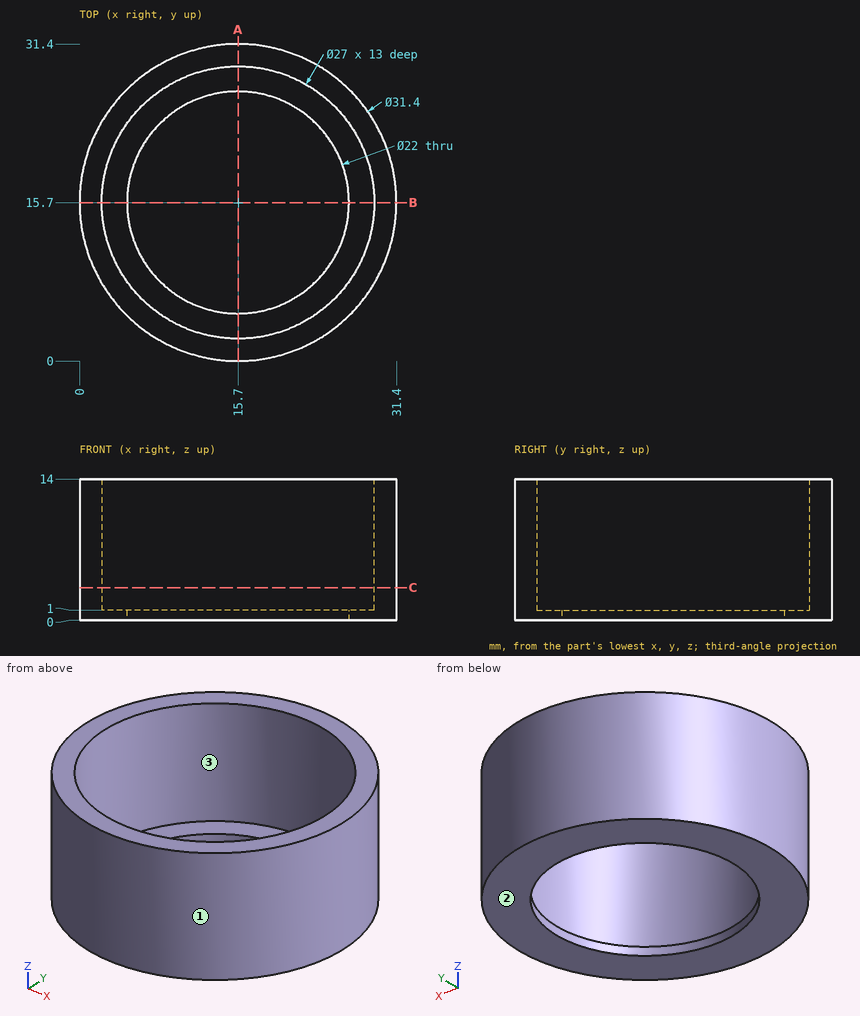
Job drawing, mm, ordinate dimensions from the low corner. One solid piece. Give positions to 0.01 mm unless a question says otherwise; leave off trailing zeros. Order: outer loops, then holes, each group sorted by start corner. A loop starts at its lowest first (then second) coordinate and runs counter-clockwise, first axis right, second up. Notation, with made-up numbers: (29, 10) - (62, 10) arc R15 ccw to (62, 17) - close; hole circle Ø4 at (68, -7). An arc over 180 degrees is marked (long way). Return JSON: item names as keys, results as strings.
1) Cut at C-C, the plane z = 3.25. Give the cut face in (x, y), plus the area to 3 significant figures.
Geometry says:
{"outline": "circle Ø31.4 at (15.7, 15.7); hole circle Ø27 at (15.7, 15.7)", "area": "202 mm²"}
2) Cut at A-A, the plane x = 15.7. Give the cut face in (y, z).
Geometry says:
{"outline": "(0, 0) - (4.7, 0) - (4.7, 1) - (2.2, 1) - (2.2, 14) - (0, 14) - close; (26.7, 0) - (31.4, 0) - (31.4, 14) - (29.2, 14) - (29.2, 1) - (26.7, 1) - close"}
3) Probe line 1 (Y direction, x = 15.7, z = 0.2); line 2 (X direction, y = 16, z = 1.25); line 3 (Y direction, x = 24, z = 13). List the from-to ranges inside material, lowest first. Write a range as from..to.
Geometry says:
{"line 1": "0..4.7, 26.7..31.4", "line 2": "0..2.2, 29.2..31.4", "line 3": "2.37..5.05, 26.35..29.03"}
4) Flat gauge pins, fed straight in: P1, Ø1, axis at x = 6, z = 2, coming from the +Y side; P2, Ø3, axis at x = 18, z = 7.5, coming from the +Y side; P3, Ø3, axis at x = 3.5, z = 2.5, coming from the +Y side. Where does each tip first touch, or does it go through?
Geometry says:
{"P1": "y = 28.42", "P2": "y = 31.38", "P3": "y = 27.19"}
5) Pull direction Y, two halves, no side cores. Call the marked faces 1, 2 and 3: pulls with the +Y half, pulls with the -Y half, needs draft (parallel to the pull), parting line crosses it, or undercut.
Geometry says:
{"face 1": "parting line crosses it", "face 2": "needs draft", "face 3": "undercut"}
